from build123d import *

# Parameters (mm, degrees)
F1_DEPTH = 0.6096
F2_W     = 0.6096
F2_H     = 0.6096
F3_DEPTH = 4.7625
F5_DEPTH = 4.7625


with BuildPart() as f1:
    # F0 (on Front) → F1 (new body)
    with BuildSketch(Plane.XZ):
        with BuildLine():
            Line((-37.084, 0), (0, 0))
            Line((0, 0), (0, 0.79375))
            ThreePointArc((0, 0.79375), (-18.542, 4.000644), (-37.084, 0.79375))
            Line((-37.084, 0.79375), (-37.084, 0))
        make_face()
    extrude(amount=-F1_DEPTH)

    # F2 (on face) → F3 (join)
    with BuildSketch(Plane.XZ):
        Polygon((-37.084, 0.6096), (-37.084, 0), (-36.8046, 0), (-36.195, 0), (-36.184512, 0.6096), align=None)
        with Locations((-36.4998, -0.3048)):
            Rectangle(F2_W, F2_H)
        with Locations((-0.5842, -0.3048)):
            Rectangle(F2_W, F2_H)
        Polygon((-0.889, 0.6096), (-0.889, 0), (-0.2794, 0), (0, 0), (0, 0.6096), align=None)
    extrude(amount=F3_DEPTH)

    # F4 (on face) → F5 (join)
    with BuildSketch(Plane.XZ):
        with BuildLine():
            Line((-0.889, 0), (-0.889, 0.6096))
            ThreePointArc((-0.889, 0.6096), (-18.536756, 3.338909), (-36.184512, 0.6096))
            Line((-36.184512, 0.6096), (-36.195, 0))
            Line((-36.195, 0), (-36.000362, 0.02848))
            ThreePointArc((-36.000362, 0.02848), (-18.536756, 2.729309), (-1.07315, 0.02848))
            Line((-1.07315, 0.02848), (-0.889, 0))
        make_face()
    extrude(amount=F5_DEPTH)


solid = f1.part
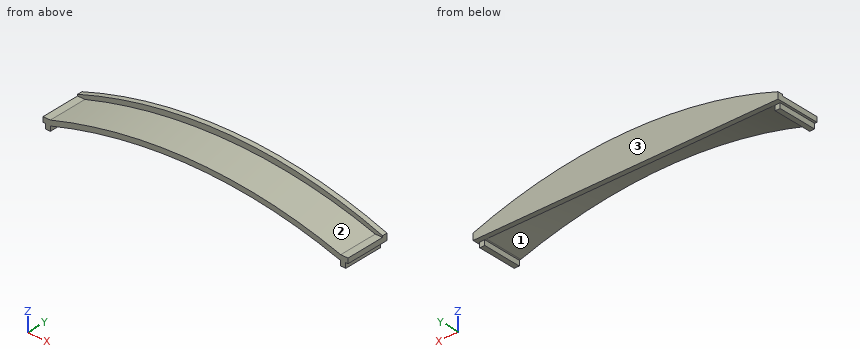
Could you check a few things on this model? Use its own coordinates, in mm. Face numbers are marked on the shaded views. Give positions to 0.01 mm unless a question says otherwise; leave off trailing zeros. Order: outer loops, then holes, each group sorted by start corner. A loop starts at its lowest first (then second) coordinate and runs counter-clockwise, first axis right, second up.
Item 1: I need wall thicknesses on line 1 (X direction, y = -4.15, z = -0.05) (3 decimals); line 2 (Y direction, x = -17.5, z = 2.5); line 3 (Z direction, x = -14, y = -2.9). Which ranges of each line are inside material? Lowest first, please.
Item 2: If we section it at D-D, the plane x = -25: Write out the boundary of the cut face in (y, z), plus the area to 3 significant figures.
Item 3: If we section it at B-B, the plane x = -6.5: Write out the boundary of the cut face in (y, z).
Item 4: I'm going to push flat-ended pins straight in: pin 1 (2 mm diameter, centred on y = -2.5, z = 1.5, fed in from +X); pin 2 (2.5 mm diameter, centred on x = -17, y = -2.5, fed in from -Z); pin 3 (0.7 mm diameter, centred on x = -36.5, z = -0.5, fed in from +Y); pin 4 (0.7 mm diameter, centred on y = -2, z = -0.5, fed in from -X). Where does each tip first touch, or does it pass through?
Item 5: If we section it at A-A, the plane y = -3.4: Write out the boundary of the cut face in (x, z) (3 decimals), plus the area to 3 significant figures.
Item 6: If we mould it in two halves opening along X, with no side actions, what happens to the marked faces 1, 2 and 3? For each: pulls with the +X half, pulls with the -X half, needs draft (parallel to the pull), parting line crosses it, or undercut.
Item 7: If we section it at C-C, the plane z = 1.3: Write out the boundary of the cut face in (x, y), plus the area to 3 significant figures.
Values:
1. line 1: x = -36.805 to -36.195, -0.889 to -0.279
1. line 2: y = 0 to 0.61
1. line 3: z = 2.55 to 3.16
2. outline: (-4.76, 2.37) - (0, 2.37) - (0, 0) - (0.61, 0) - (0.61, 3.62) - (0, 3.62) - (0, 2.98) - (-4.76, 2.98) - close
2. area: 5.13 mm2
3. outline: (-4.76, 1.46) - (0, 1.46) - (0, 0) - (0.61, 0) - (0.61, 2.67) - (0, 2.67) - (0, 2.09) - (-4.76, 2.09) - close
4. pin 1: stops at x = 0
4. pin 2: stops at z = 2.66
4. pin 3: stops at y = 0
4. pin 4: stops at x = -36.8
5. outline: (-37.084, 0) - (-36.805, 0) - (-36.805, -0.61) - (-36.195, -0.61) - (-36.195, 0) - (-36, 0.028) arc R57.81 cw to (-1.073, 0.028) - (-0.889, 0) - (-0.889, -0.61) - (-0.279, -0.61) - (-0.279, 0) - (0, 0) - (0, 0.61) - (-0.889, 0.61) arc R58.42 ccw to (-36.185, 0.61) - (-37.084, 0.61) - close
5. area: 23.7 mm2
6. face 1: undercut
6. face 2: parting line crosses it
6. face 3: needs draft
7. outline: (-35.6, 0) - (-33.84, 0) - (-33.84, -4.76) - (-31.31, -4.76) - (-31.31, 0) - (-5.76, 0) - (-5.76, -4.76) - (-3.24, -4.76) - (-3.24, 0) - (-1.49, 0) - (-1.49, 0.61) - (-35.6, 0.61) - close
7. area: 44.8 mm2
